The listing builds one solid part. Answer for the finished solid, in the listing's coordinates (mm). Round coordinates to 2 decimals unless told otherwise and drop trailing zeros. Loops run counter-clockwise (first coordinate to the right, second up) from the corner with the lowest first, then second, coordinate; pieces in that order, holes last. Notation, with made-up numbers: M 32.5,37 L 70.5,37 A31 cw 70.5,67 Z; hole C -13.75,38 d7. An arc over 180 degrees is marked long. Answer as a JSON object with one key per item and string values.
```python
from build123d import *

# Parameters (mm, degrees)
SKETCH_1_W          = 4
SKETCH_1_H          = 20
EXTRUDE_1_DEPTH     = 4
SKETCH_2_W          = 70.761600996
SKETCH_2_H          = 28.517073099
CUT_EXTRUDE_1_DEPTH = 4
SKETCH_3_W          = 69.96653911
SKETCH_3_H          = 17
CUT_EXTRUDE_2_DEPTH = 10


with BuildPart() as part:
    # Эскиз1 → Бобышка-Вытянуть1 (new body)
    with BuildSketch(Plane.XY):
        with Locations((-52.9, -10)):
            Rectangle(SKETCH_1_W, SKETCH_1_H)
        with Locations((-52.9, -50)):
            Rectangle(SKETCH_1_W, SKETCH_1_H)
        Polygon((0, -20), (0, 0), (-50.9, 0), (-50.9, -20), (-50.9, -40), (-50.9, -60), (-50.9, -80), (-50.9, -89.071572875), (0, -89.071572875), (0, -60), (0, -40), align=None)
        with Locations((2, -10)):
            Rectangle(SKETCH_1_W, SKETCH_1_H)
        with Locations((2, -50)):
            Rectangle(SKETCH_1_W, SKETCH_1_H)
    extrude(amount=EXTRUDE_1_DEPTH)

    # Эскиз2 → Вырез-Вытянуть1 (cut)
    with BuildSketch(Plane(origin=(0, 0, 0), x_dir=(-1, 0, 0), z_dir=(0, 0, -1))):
        with Locations((19.519199502, -5.74146345)):
            Rectangle(SKETCH_2_W, SKETCH_2_H)
    extrude(amount=-CUT_EXTRUDE_1_DEPTH, mode=Mode.SUBTRACT)

    # Эскиз3 → Вырез-Вытянуть2 (cut)
    with BuildSketch(Plane(origin=(0, 0, 0), x_dir=(-1, 0, 0), z_dir=(0, 0, -1))):
        with Locations((15.916730445, -80.571572875)):
            Rectangle(SKETCH_3_W, SKETCH_3_H)
    extrude(amount=-CUT_EXTRUDE_2_DEPTH, mode=Mode.SUBTRACT)


solid = part.part
```
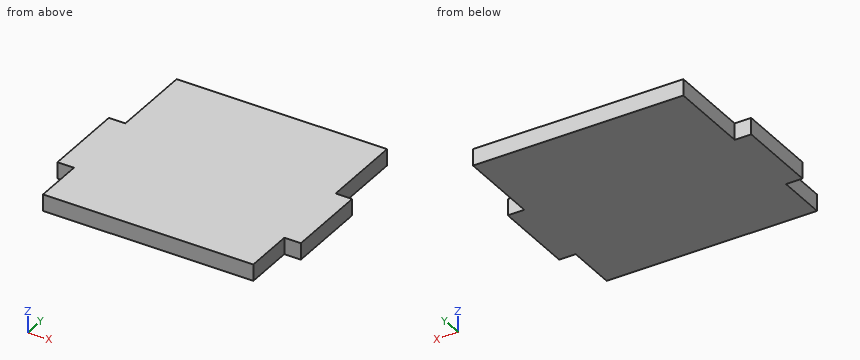
Item 1: The part is cut by section B-B (y = -63.5). Give the vertices of the cut face in (x, z), then the cut area to 3 significant figures.
Values follow:
{"outline": "M -50.9,0 L 0,0 L 0,4 L -50.9,4 Z", "area": "204 mm^2"}
Item 2: Flat-ended cylindrical pins translate along their axes: P1, Ø2, axis at x = -53.5, z = 3, coming from the +Y side; P2, Ø1.2, axis at y = -33, z = 3, coming from the +X side; P3, Ø1.2, axis at x = -52, z = 1.5, coming from the -Y side. Find the tip coordinate at first contact, or state that the pin passes through.
Values follow:
{"P1": "y = -40", "P2": "x = 0", "P3": "y = -60"}
Item 3: The part is cut by section A-A (z = 2). Give the vertices of the cut face in (x, y), then the cut area to 3 significant figures.
Values follow:
{"outline": "M -54.9,-60 L -50.9,-60 L -50.9,-72.07 L 0,-72.07 L 0,-60 L 4,-60 L 4,-40 L 0,-40 L 0,-20 L -50.9,-20 L -50.9,-40 L -54.9,-40 Z", "area": "2,810 mm^2"}
Item 4: Straight lines are drawn through the part: line 1 (X direction, y = -64.5, z = 1.05); line 2 (Y direction, x = -51, z = 0.6). For each, find the intervals that lie inside material, in ascending order.
Values follow:
{"line 1": "-50.9 to 0", "line 2": "-60 to -40"}
